Check sheet for the modelled part. Datum: model origin and axes. Units: mm. Face numbers are marked on the shaded views. A direction names the side the tool comes from. Round coordinates to 2 decimals unless told otherwise and drop trailing zeros. Write each loop counter-clockwise with the first axis right and the second up, starting at its lowest first coordinate (ties: lowest second). Pieces come first, ordered by that corner, then holes.
Item 1: Section check D-D, the plane z = 8.5. Record the cut outline in (x, y), plus the area to 3 significant figures.
Item 2: Section check A-A, the plane z = -3. Record the cut outline in (x, y).
Item 3: Section check B-B, the plane y = -44.25. Record the cut outline in (x, z).
Item 4: Depth check by flat-ended pin: pin 1 (3.5 mm diameter, centred on x = -13, y = -43, fed in from -Z); pin 2 (5 mm diameter, centred on y = -49, z = 3, fed in from +X); pin 3 (6 mm diameter, centred on y = -43.5, z = 3.5, fed in from +X); pin 4 (4 mm diameter, centred on x = -8.5, z = -3, fed in from +Y). Enter the tip coordinate at first touch or a pass-through.
Item 5: Material ranges on line 1 along X through (y, z) = (-43.5, 6.25); line 2 along Z through (x, y) = (-12.25, -45.25); line 3 along Z through (x, y) = (-5.75, -46), recorded low to high.
Item 6: Release check for a two-part mould opening along Y. For the marked faces 3, 4, 5 and 6 record: pulls with the +Y half, pulls with the -Y half, needs draft (parallel to the pull), parting line crosses it, or undercut.
Item 7: Section check C-C, the plane z = 5.5. Record the cut outline in (x, y), plus the area to 3 significant figures.
Item 8: Set-up check for the marked faces 1 and 2: record each of +Z, -Z, +X, -X, +Y, -Y from which the full face is reachable in a straight line by a thin tool's end or side.
from build123d import *

# Parameters (mm, degrees)
EXTRUSION1_DEPTH = 8
ESQUISSE2_R      = 1.15
EXTRUSION2_DEPTH = 1.2
EXTRUSION3_START = 5
EXTRUSION3_DEPTH = 5


with BuildPart() as part:
    # Esquisse1 → Extrusion1 (new body)
    with BuildSketch(Plane.XY):
        with BuildLine():
            Line((-14.760065323, -47.656078111), (-4.714170639, -41.856078111))
            ThreePointArc((-4.714170639, -41.856078111), (-4.178355938, -41.157790798), (-4.293241424, -40.285148896))
            Line((-4.293241424, -40.285148896), (-6.718241424, -36.084925688))
            Line((-6.718241424, -36.084925688), (-10.528753201, -38.284925688))
            Line((-10.528753201, -38.284925688), (-7.778753201, -43.048065409))
            Line((-7.778753201, -43.048065409), (-11.675867518, -45.298065409))
            Line((-11.675867518, -45.298065409), (-14.425867518, -40.534925688))
            Line((-14.425867518, -40.534925688), (-18.755994537, -43.034925688))
            Line((-18.755994537, -43.034925688), (-16.330994537, -47.235148896))
            ThreePointArc((-16.330994537, -47.235148896), (-15.632707224, -47.770963597), (-14.760065323, -47.656078111))
        make_face()
    extrude(amount=EXTRUSION1_DEPTH)

    # Esquisse2 → Extrusion2 (add)
    with BuildSketch(Plane.XY.offset(8)):
        Polygon((-18.755994537, -43.034925688), (-16.330994537, -47.235148896), (-13.255994537, -52.56120513), (-1.218241424, -45.61120513), (-4.293241424, -40.285148896), (-6.718241424, -36.084925688), (-10.528753201, -38.284925688), (-7.778753201, -43.048065409), (-11.675867518, -45.298065409), (-14.425867518, -40.534925688), align=None)
        with Locations((-8.412117981, -47.051045431)):
            Circle(ESQUISSE2_R, mode=Mode.SUBTRACT)
    extrude(amount=EXTRUSION2_DEPTH)

    # Esquisse3 → Extrusion3 (add)
    with BuildSketch(Plane(origin=(0, 0, 0), x_dir=(-1, 0, 0), z_dir=(0, 0, -1)).offset(EXTRUSION3_START)):
        with BuildLine():
            ThreePointArc((4.714170639, -41.856078111), (5.864170639, -41.856078111), (6.439170639, -40.860148896))
            ThreePointArc((6.439170639, -40.860148896), (5.586812541, -39.749334196), (4.293241424, -40.285148896))
            ThreePointArc((4.293241424, -40.285148896), (4.178355938, -41.157790798), (4.714170639, -41.856078111))
        make_face()
        with BuildLine():
            ThreePointArc((16.330994537, -47.235148896), (16.445880023, -46.957790798), (16.485065323, -46.660148896))
            ThreePointArc((16.485065323, -46.660148896), (14.760065323, -45.664219682), (14.760065323, -47.656078111))
            ThreePointArc((14.760065323, -47.656078111), (15.632707224, -47.770963597), (16.330994537, -47.235148896))
        make_face()
    extrude(amount=-EXTRUSION3_DEPTH)


solid = part.part
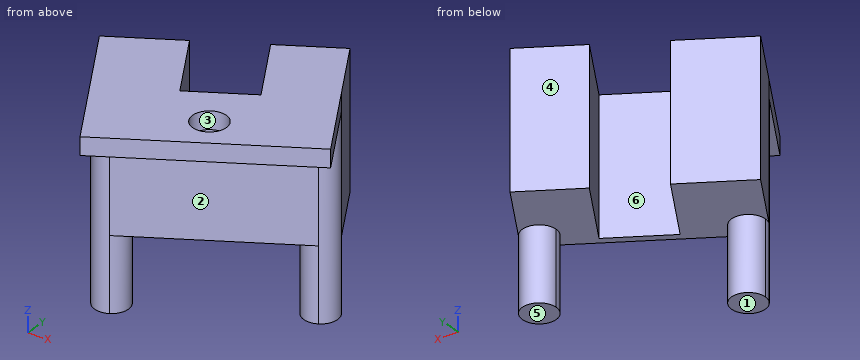
Values found:
1. outline: (-18.76, -43.03) - (-13.26, -52.56) - (-1.22, -45.61) - (-6.72, -36.08) - (-10.53, -38.28) - (-7.78, -43.05) - (-11.68, -45.3) - (-14.43, -40.53) - close; hole circle Ø2.3 at (-8.41, -47.05)
1. area: 124 mm2
2. outline: circle Ø2.3 at (-15.34, -46.66); circle Ø2.3 at (-5.29, -40.86)
3. outline: (-18.05, 0) - (-12.28, 0) - (-12.28, 9.2) - (-18.05, 9.2) - close; (-9.86, 0) - (-8.86, 0) - (-8.86, 8) - (-2, 8) - (-2, 9.2) - (-9.86, 9.2) - close
4. pin 1: stops at z = 0
4. pin 2: stops at x = -12.76
4. pin 3: stops at x = -4.14
4. pin 4: passes through
5. line 1: x = -18.49 to -12.71, -8.56 to -7.56
5. line 2: z = 0 to 9.2
5. line 3: z = 8 to 9.2
6. face 3: undercut
6. face 4: pulls with the +Y half
6. face 5: needs draft
6. face 6: undercut
7. outline: (-18.76, -43.03) - (-16.33, -47.24) arc R1.15 ccw to (-14.76, -47.66) - (-4.71, -41.86) arc R1.15 ccw to (-4.29, -40.29) - (-6.72, -36.08) - (-10.53, -38.28) - (-7.78, -43.05) - (-11.68, -45.3) - (-14.43, -40.53) - close
7. area: 58.1 mm2
8. face 1: -Z, +X, -X, +Y, -Y
8. face 2: -Z, +X, -Y
